Autodesk Inventor part; units mm, degrees
ref_plane "РабПлоскость1" through (0, 0, 19) normal (0, 0, 1) x (1, 0, 0)
ref_plane "РабПлоскость2" through (0, 0, 25.5) normal (0, 0, 1) x (1, 0, 0)
ref_plane "YZ Plane" through (0, 0, 0) normal (1, 0, 0) x (0, 1, 0)
sketch "Эскиз1" plane through (0, 0, 0) normal (0, 0, 1) x (1, 0, 0)
  line L0 (0, 0) -> (761, 0)
  line L1 (0, 0) -> (0, 25)
  line L2 (0, 25) -> (90, 25)
  line L3 (90, 25) -> (90, 27.5)
  line L4 (90, 27.5) -> (131, 27.5)
  line L5 (131, 27.5) -> (131, 30)
  line L6 (425.5, 30) -> (425.5, 0) construction
  line L7 (720, 27.5) -> (720, 30)
  line L8 (131, 30) -> (148, 30)
  line L9 (148, 30) -> (148, 32.5)
  line L10 (148, 32.5) -> (181, 32.5)
  line L11 (720, 30) -> (703, 30)
  line L12 (703, 30) -> (703, 32.5)
  line L13 (703, 32.5) -> (181, 32.5)
  line L14 (720, 27.5) -> (761, 27.5)
  line L15 (761, 27.5) -> (761, 0)
  dimension "d0" = 50
  dimension "d1" = 55
  dimension "d2" = 90
  dimension "d3" = 41
  dimension "d14" = 17
  dimension "d15" = 60
  dimension "d16" = 65
  dimension "d27" = 41
  dimension "d29" = 630
revolve "Вращение1" add sketch "Эскиз1" angle 360 about axis through (0, 0, 0) along (1, 0, 0)
ref_plane "РабПлоскость1" through (0, 0, 19) normal (0, 0, 1) x (1, 0, 0)
sketch "Эскиз2" plane through (0, 0, 19) normal (0, 0, 1) x (1, 0, 0)
  line L0 (65, 8) -> (20, 8)
  line L1 (20, 8) -> (20, -8)
  line L2 (20, -8) -> (65, -8)
  line L3 (65, -8) -> (65, 8)
  arc A0 (65, -8) -> (65, 8) centre (65, 0) ccw
  arc A1 (20, 8) -> (20, -8) centre (20, 0) ccw
  point P0 (0, 0)
  dimension "d8" = 8
  dimension "d9" = 16
  dimension "d10" = 45
  dimension "d11" = 20
extrude "Выдавливание1" cut sketch "Эскиз2" along normal blind 33
ref_plane "РабПлоскость2" through (0, 0, 25.5) normal (0, 0, 1) x (1, 0, 0)
sketch "Эскиз3" plane through (0, 0, 25.5) normal (0, 0, 1) x (1, 0, 0)
  line L0 (148, -32.5) -> (148, 32.5)
  line L1 (400.5, 9) -> (450.5, 9)
  line L2 (450.5, 9) -> (450.5, -9)
  line L3 (450.5, -9) -> (400.5, -9)
  line L4 (400.5, -9) -> (400.5, 9)
  arc A0 (400.5, 9) -> (400.5, -9) centre (400.5, 0) ccw
  arc A1 (450.5, -9) -> (450.5, 9) centre (450.5, 0) ccw
  line L5 (703, -30) -> (703, 30)
  point P0 (0, 0)
  dimension "d19" = 18
  dimension "d20" = 252.5
  dimension "d21" = 50
  dimension "d22" = 9
  dimension "d26" = 555
extrude "Выдавливание2" cut sketch "Эскиз3" along normal blind 44.75
chamfer "Фаска1" distance 2 angle 45 1 edges at (0, -25, 0)
equation "\"d27\" = d3"
properties part number "Валл" material "Сталь, углеродистая"
Could you check a few things on this model? Use its own coordinates, in mm. A direction names the side the tool comes from. Coordinates: 2 decimals unless noted, no trailing zeros. Loops run counter-clockwise (first coordinate to the right, second up) from the corner with the lowest first, then second, coordinate; pieces in that order, holes last.
1. We'd pull the mould along X, two halves only. Please class faces 1 (the face through (0.125, -18.351, -14.071)), 2 (the face through (42, 0, 19)), 3 (the face through (711.38, -29.97, -1.32)): released by +X, released by -X, zero draft, split by the parting line, or undercut.
2. Imagine slicing it at B-B (z = 0). Please give me the cut outline in (x, y).
3. I need wall thicknesses on L1, parallel to X at y = 21.5, z = 16; L2, parallel to Z at x = 620, y = -1.5; L3, parallel to Y at x = 659, z = 8. Which ranges of each line are inside material? Lowest first, please.
4. For faces 4 (the face through (720, 13.2, -24.3)), 5 (the face through (131, 13.2, -24.3)), 6 (the face through (0, 0, 0)), 7 (the face through (761, 0, 0)), 8 (the face through (425, 0, 25.5)), which set-ups out of +Z, -Z, +X, -X, +Y, -Y let a thin tool reach every point of the face, with its end or its side?
5. For P1, Ø6.5, axis at x = 434, z = 28.5, coming from the -Y side; P2, Ø1.7, axis at x = 424.5, z = 28, coming from the +Y side; P3, Ø8, axis at x = 339, y = 24, coming from the -Z side, each with a flat end and sliding along its axis, tell me the tip position at first contact or that it passes through.
6. Imagine slicing it at C-C (x = 182). Please give me the cut outline in (y, z), and give its area (3 significant figures).
Computed values:
1. face 1: released by -X
1. face 2: undercut
1. face 3: zero draft
2. outline: (0, -23) - (2, -25) - (90, -25) - (90, -27.5) - (131, -27.5) - (131, -30) - (148, -30) - (148, -32.5) - (703, -32.5) - (703, -30) - (720, -30) - (720, -27.5) - (761, -27.5) - (761, 27.5) - (720, 27.5) - (720, 30) - (703, 30) - (703, 32.5) - (148, 32.5) - (148, 30) - (131, 30) - (131, 27.5) - (90, 27.5) - (90, 25) - (2, 25) - (0, 23) - close
3. L1: x = 90 to 761
3. L2: z = -32.47 to 32.47
3. L3: y = -31.5 to 31.5
4. face 4: +X
4. face 5: -X
4. face 6: +Z, -Z, -X, +Y, -Y
4. face 7: +Z, -Z, +X, +Y, -Y
4. face 8: +Z
5. P1: stops at y = -20.46
5. P2: stops at y = 17.86
5. P3: stops at z = -25.62
6. outline: circle Ø65 at (0, 0)
6. area: 3,320 mm2
